Work out the finished part from the listing and answer in its coordinate system (mm). Give positions to 0.01 mm unless a question says otherwise; leave off trailing zeros. Order: outer loops, then holes, each group sorted by start corner. A loop starts at its lowest first (then second) coordinate and runs counter-clockwise, first axis right, second up.
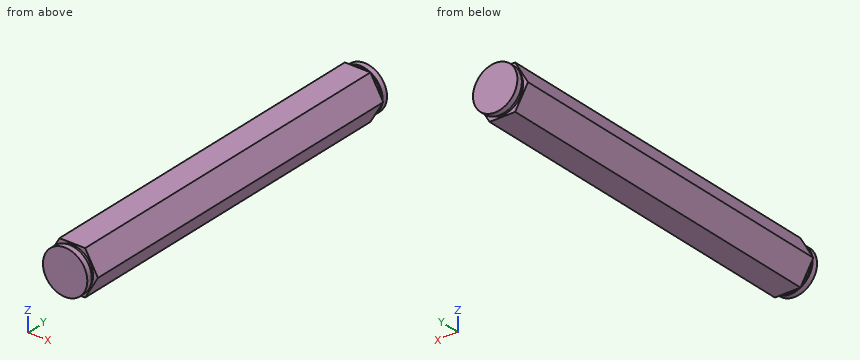
```python
from build123d import *

# Parameters (mm, degrees)
F1_DEPTH      = 51.196875
F1_DEPTH_BACK = 51.196875
F2_R          = 5.9436
F3_DEPTH      = 0.9906
F4_R          = 6.35
F5_DEPTH      = 1.5875


# Not quite as in the source:
# - a pattern or mirror of a feature is missing from the dataset's text; its kind, count and spacing are read off the source's solid


with BuildPart() as f1:
    # F0 (on Front) → F1 (new body, two sides)
    with BuildSketch(Plane.XZ) as f1_sk:
        Polygon((3.6661742094, 6.35), (-3.6661742094, 6.35), (-7.3323484187, 0), (-3.6661742094, -6.35), (3.6661742094, -6.35), (7.3323484187, 0), align=None)
    extrude(amount=F1_DEPTH)
    extrude(f1_sk.sketch, amount=-F1_DEPTH_BACK)

    # F2 (on face) → F3 (join)
    with BuildSketch(Plane.XZ.offset(51.196875)):
        Circle(F2_R)
    f3 = extrude(amount=F3_DEPTH)

    # F3_copies: F3 across plane
    add(f3.mirror(Plane.ZX))

    # F4 (on face) → F5 (join)
    with BuildSketch(Plane.XZ.offset(52.187475)):
        Circle(F4_R)
    f5 = extrude(amount=F5_DEPTH)

    # F5_copies: F5 across plane
    add(f5.mirror(Plane.ZX))


solid = f1.part
```
1. The part is cut by section B-B (y = -0.5). Write down the section's boundary in (x, z), then the cut area to 3 significant figures.
Findings below:
outline: (-7.33, 0) - (-3.67, -6.35) - (3.67, -6.35) - (7.33, 0) - (3.67, 6.35) - (-3.67, 6.35) - close
area: 140 mm2
2. The part is cut by section A-A (z = -2). Write down the section's boundary in (x, y), then the cut area to 3 significant figures.
Findings below:
outline: (-6.18, -51.2) - (-5.6, -51.2) - (-5.6, -52.19) - (-6.03, -52.19) - (-6.03, -53.77) - (6.03, -53.77) - (6.03, -52.19) - (5.6, -52.19) - (5.6, -51.2) - (6.18, -51.2) - (6.18, 51.2) - (5.6, 51.2) - (5.6, 52.19) - (6.03, 52.19) - (6.03, 53.77) - (-6.03, 53.77) - (-6.03, 52.19) - (-5.6, 52.19) - (-5.6, 51.2) - (-6.18, 51.2) - close
area: 1,330 mm2
3. Given P1, Ø5, axis at x = 5, y = 34.5, coming from the -Z side; P2, Ø4, axis at y = 36, z = -3, coming from the +X side (3 decimals); P3, Ø3, axis at y = 24.5, z = 2, coming from the -X side, each flat-ended and moving along its own axis, determine where each tip first touches the part or whether it passes through.
Findings below:
P1: stops at z = -6.35
P2: stops at x = 6.755
P3: stops at x = -7.04
4. The part is cut by section C-C (z = 2.5). Write down the section's boundary in (x, y).
Findings below:
outline: (-5.89, -51.2) - (-5.39, -51.2) - (-5.39, -52.19) - (-5.84, -52.19) - (-5.84, -53.77) - (5.84, -53.77) - (5.84, -52.19) - (5.39, -52.19) - (5.39, -51.2) - (5.89, -51.2) - (5.89, 51.2) - (5.39, 51.2) - (5.39, 52.19) - (5.84, 52.19) - (5.84, 53.77) - (-5.84, 53.77) - (-5.84, 52.19) - (-5.39, 52.19) - (-5.39, 51.2) - (-5.89, 51.2) - close
5. Straight lines are drawn through the part: probe 1 along X at (y, z) = (-35, -1.75); probe 2 along X at (y, z) = (4.5, -3). For each, find the intervals that lie inside material, in ascending order.
Findings below:
probe 1: x = -6.32 to 6.32
probe 2: x = -5.6 to 5.6
